Autodesk Inventor part; units mm, degrees
ref_plane "YZ Plane" through (0, 0, 0) normal (1, 0, 0) x (0, 1, 0)
ref_plane "XZ Plane" through (0, 0, 0) normal (0, 1, 0) x (-1, 0, 0)
ref_plane "XY Plane" through (0, 0, 0) normal (0, 0, 1) x (1, 0, 0)
sketch "Sketch1" plane through (0, 0, 0) normal (0, 1, 0) x (-1, 0, 0)
  circle A0 centre (0, 0) radius 14
  circle A1 centre (0, 0) radius 7.5
  dimension "d0" = 28
  dimension "d1" = 15
extrude "Extrusion1" add sketch "Sketch1" along normal blind 7
sketch "Sketch2" plane through (0, 7, 0) normal (0, 1, 0) x (1, 0, 0)
  line L0 (14, -3.75) -> (-14, -3.75)
  line L1 (-14, -3.75) -> (-14, 3.75)
  line L2 (-14, 3.75) -> (14, 3.75)
  line L3 (14, 3.75) -> (14, -3.75)
  line L4 (14, -3.75) -> (-14, 3.75) construction
  line L5 (-14, -3.75) -> (14, 3.75) construction
  line L6 (-0.5, 5) -> (0.5, 5)
  line L7 (0.5, 5) -> (0.5, -5)
  line L8 (0.5, -5) -> (-0.5, -5)
  line L9 (-0.5, -5) -> (-0.5, 5)
  line L10 (-0.5, 5) -> (0.5, -5) construction
  line L11 (0.5, 5) -> (-0.5, -5) construction
  circle A0 centre (0, 0) radius 7.5
  circle A1 centre (0, 0) radius 14
  point P0 (0, 0)
  point P1 (-13.4884, 3.75)
  point P2 (-13.4884, -3.75)
  point P3 (-6.4952, -3.75)
  point P4 (-6.4952, 3.75)
  point P5 (13.4884, 3.75)
  point P6 (6.4952, 3.75)
  point P7 (6.4952, -3.75)
  point P8 (13.4884, -3.75)
  dimension "d4" = 28
  dimension "d5" = 7.5
  dimension "d27" = 15
  dimension "d28" = 28
sketch "Sketch3" plane through (0, 0, 0) normal (0, -1, 0) x (1, 0, 0)
  circle A0 centre (0, 0) radius 14
  dimension "d17" = 28
extrude "Extrusion3" add sketch "Sketch3" along normal blind 2
sketch "Sketch5" plane through (0, 0, 0) normal (0, 1, 0) x (1, 0, 0)
  point P0 (0, 0)
  point P1 (-0.0372, -0.1116)
hole "Hole2" at (-0.0372, 0, 0.1116) direction (0, -1, 0) diameter 4.5 end through all
extrude "Extrusion4" add sketch "Sketch2" along normal blind 4.5 contours L0 A0 L2 A1 | A1 L2 A0 L0
properties part number "magneticslotV1"
Model file for the job. Use its own axes, mm. A direction names the side the tool comes from. Round coordinates to 2 decimals unless told otherwise and drop trailing zeros. Loops run counter-clockwise (first coordinate to the right, second up) from the corner with the lowest first, then second, coordinate; pieces in that order, holes last. Notation, with made-up numbers: (-19, 67.25) - (21, 67.25) arc R29 cw to (21, 102.25) - close; hole circle Ø8 at (66, 42). An arc over 180 degrees is marked (long way). Write each question's results on one line, items separated by ' | '.
(1) Saw through at B-B, the plane z = 0. List the corners of the cut face in (x, y), then the cut area to 3 significant figures.
Answer below:
outline: (-14, -2) - (-2.28, -2) - (-2.28, 0) - (-7.5, 0) - (-7.5, 11.5) - (-14, 11.5) - close; (2.21, -2) - (14, -2) - (14, 11.5) - (7.5, 11.5) - (7.5, 0) - (2.21, 0) - close | area: 197 mm^2
(2) Saw through at C-C, the plane y = 3.5. List the corners of the cut face in (x, z).
Answer below:
outline: circle Ø28 at (0, 0); hole circle Ø15 at (0, 0)
(3) Saw through at A-A, the plane y = 8.25. List the corners of the cut face in (x, z).
Answer below:
outline: (-13.49, -3.75) - (-6.5, -3.75) arc R7.5 cw to (-6.5, 3.75) - (-13.49, 3.75) arc R14 ccw to start; (6.5, -3.75) - (13.49, -3.75) arc R14 ccw to (13.49, 3.75) - (6.5, 3.75) arc R7.5 cw to start
(4) Pin check, flat tips, straight feed: pin 1 (1 mm diameter, centred on y = 9.5, z = -1.5, fed in from -X); pin 2 (2 mm diameter, centred on y = 0.5, z = 3, fed in from -X); pin 3 (8 mm diameter, centred on x = -3.5, z = -9, fed in from +Y); pin 4 (5 mm diameter, centred on x = -2.5, y = -0.5, fed in from +Z). Stop position of each tip, or through.
Answer below:
pin 1: stops at x = -13.96 | pin 2: stops at x = -13.86 | pin 3: stops at y = 7 | pin 4: stops at z = 14
(5) Saw through at D-D, the plane x = -3.25. List the corners of the cut face in (y, z), then the cut area to 3 significant figures.
Answer below:
outline: (-2, -13.62) - (7, -13.62) - (7, -6.76) - (0, -6.76) - (0, 6.76) - (7, 6.76) - (7, 13.62) - (-2, 13.62) - close | area: 150 mm^2
(6) Wall check: L1, parallel to X at y = 7.25, z = 0; L2, parallel to Y at x = -6.25, z = -0.25; L3, parallel to Y at x = 10.75, z = 5. Give the ranges that are in metal, low to high.
Answer below:
L1: x = -14 to -7.5, 7.5 to 14 | L2: y = -2 to 0 | L3: y = -2 to 7
(7) 3-axis set-ups, long thin cutter, end or side, ignore diameter. For faces 1 (the flat face through (0, -2, -3)), 2 (the cylindrical face through (-2.84, 4.39, 6.94)), 3 (the flat face through (0, 7, -9)), 4 (the flat face through (0, 7, 9)): which of +Z, -Z, +X, -X, +Y, -Y reach the whole face in a straight line?
Answer below:
face 1: +Z, -Z, +X, -X, -Y | face 2: +Y | face 3: -Z, +X, -X, +Y | face 4: +Z, +X, -X, +Y
(8) Mould opens along Z. For faces 5 (the flat face through (10, 9, -3.75)), 6 (the flat face through (2, 0, -2)), 7 (the flat face through (10, 11.5, 0)) say: released by +Z, released by -Z, zero draft, split by the parting line, or undercut.
Answer below:
face 5: released by -Z | face 6: undercut | face 7: zero draft
